The figure shows three views and two pictorial views of one solid part (mm, origin at its lowest corner). Answer the questions. A direction names the side the tool comes from. Give positions to 0.01 mm unless a question says otherwise; leave off trailing zeros. Order: outer loops, then holes, each group sorted by start corner. A loop starts at its lowest first (then second) coordinate and runs counter-clockwise, first axis right, second up. Notation, with made-up numbers: (-24, -24) - (29, -24) arc R29 cw to (29, -3) - close; hole circle Ø8 at (-8.5, -10). An arc over 180 degrees is marked (long way). Write item = value, one per line.
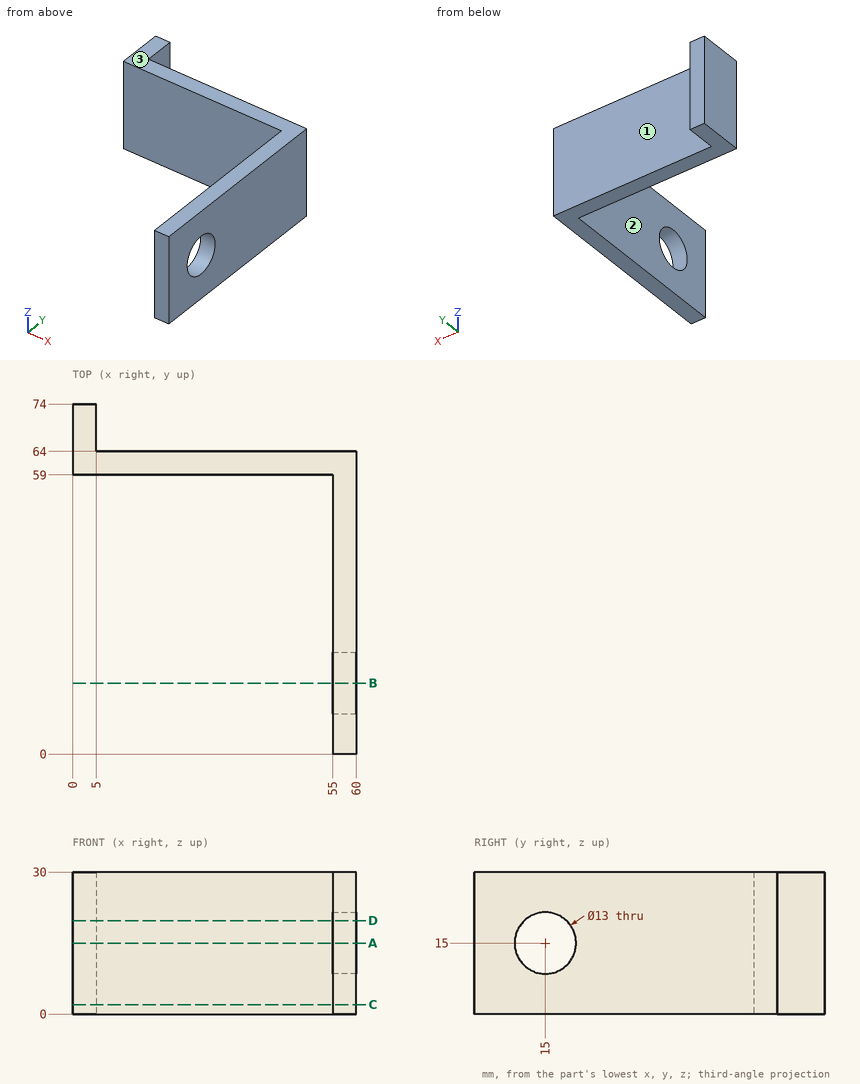
1. For the marked faces 1, 2 and 3, determine the directions among +Z, -Z, +X, -X, +Y, -Y from which every point of the face is accessible in a straight line to the end or side of a thin tool.
Recorded:
face_1 = +Z, -Z, +X, +Y
face_2 = +Z, -Z, -X, -Y
face_3 = +Z, +X, -X, +Y, -Y
2. Section A-A (z = 15) is taken. Determine the outline of the cut face in (x, y), and give its area (3 significant figures).
Recorded:
outline = (0, 59) - (55, 59) - (55, 21.5) - (60, 21.5) - (60, 64) - (5, 64) - (5, 74) - (0, 74) - close; (55, 0) - (60, 0) - (60, 8.5) - (55, 8.5) - close
area = 580 mm^2
3. Flat-ended cylindrical pins translate along their axes: pin 1 (2 mm diameter, centred on y = 56, z = 17.5, fed in from -X); pin 2 (12 mm diameter, centred on x = 52, z = 3.5, fed in from +Y); pin 3 (8 mm diameter, centred on y = 67.5, z = 13.5, fed in from +X). Find the tip coordinate at first contact, or state that the pin passes through.
Recorded:
pin_1 = 55
pin_2 = 64
pin_3 = 60
4. Section D-D (z = 19.75) is taken. Determine the outline of the cut face in (x, y).
Recorded:
outline = (0, 59) - (55, 59) - (55, 19.44) - (60, 19.44) - (60, 64) - (5, 64) - (5, 74) - (0, 74) - close; (55, 0) - (60, 0) - (60, 10.56) - (55, 10.56) - close
5. Section B-B (y = 15) is taken. Determine the outline of the cut face in (x, z), and give its area (3 significant figures).
Recorded:
outline = (55, 0) - (60, 0) - (60, 8.5) - (55, 8.5) - close; (55, 21.5) - (60, 21.5) - (60, 30) - (55, 30) - close
area = 85.0 mm^2
6. Section C-C (z = 2) is taken. Determine the outline of the cut face in (x, y), and give its area (3 significant figures).
Recorded:
outline = (0, 59) - (55, 59) - (55, 0) - (60, 0) - (60, 64) - (5, 64) - (5, 74) - (0, 74) - close
area = 645 mm^2
7. Straight lines are drawn through the part: L1, parallel to Y at x = 56.2, z = 15; L2, parallel to Y at x = 56.5, z = 4.75; L3, parallel to X at y = 53, z = 10.5. For each, find the intervals that lie inside material, in ascending order. Write a range as [from, to].
Recorded:
L1 = [0, 8.5], [21.5, 64]
L2 = [0, 64]
L3 = [55, 60]
